from build123d import *

# Parameters (mm, degrees)
F0_W     = 75.653017
F0_H     = 55.848565
F1_DEPTH = 25.4
F2_SIZE  = 5.08
F4_DEPTH = 25.4


with BuildPart() as f1:
    # F0 (on Top) → F1 (new body)
    with BuildSketch(Plane.XY):
        with Locations((37.826508, 27.924283)):
            Rectangle(F0_W, F0_H)
    extrude(amount=-F1_DEPTH)

    # F2
    f2_edges = [f1.edges().sort_by_distance(p)[0] for p in [
        (0, 27.924282, 0),
        (37.826508, 0, 0),
        (75.653017, 27.924282, 0),
        (37.826508, 55.848565, 0),
    ]]
    chamfer(f2_edges, length=F2_SIZE)

    # F3 (on Top) → F4 (join)
    with BuildSketch(Plane.XY):
        Polygon((58.621187, 18.220101), (58.621187, 39.608911), (50.699413, 39.608911), (50.699413, 26.14188), (28.518412, 26.14188), (28.518412, 39.608911), (19.408364, 39.608911), (19.408364, 18.220101), align=None)
    extrude(amount=F4_DEPTH)


solid = f1.part
Verification items for the finished model (mm, model axes). A direction names the side the tool comes from. Give positions to 0.01 mm unless a question says otherwise; leave off trailing zeros. Order: outer loops, then holes, each group sorted by start corner. A loop starts at its lowest first (then second) coordinate and runs counter-clockwise, first axis right, second up. Notation, with made-up numbers: M -38,45 L -17,45 A29 cw -17,77 Z; hole C 34,13.25 d3. An arc over 180 degrees is marked long. Use one line per item in the form item = value. Start each with the question number.
Q1. Section check D-D (y = 30.5). Enter the section's corners in (x, z).
Q2. Section check C-C (z = 16.5). Enter the section's corners in (x, y), then the cut area to 3 significant figures.
Q3. Section check B-B (y = 22.5). Enter the section's corners in (x, z), then the cut area to 3 significant figures.
Q4. Go/stop test with flat-tipped pins: pin 1 Ø17 at (y, z) = (28.5, 8) entering from -X; pin 2 Ø6.5 at (y, z) = (26, 16.5) entering from +X; pin 3 Ø10 at (x, z) = (25.5, 14.5) entering from +Y. Record where each tip stops, or that it passes through.
Q5. Mould release check, pull along X, two halves, no side actions. Record for faces 1 (the flat face through (37.3, 53.27, -2.5)), 2 (the flat face through (40, 26.142, 13)), 3 (the flat face through (73.077, 27.533, -2.504)), 4 (the flat face through (50.699, 33, 13)): +X half, -X half, draft (parallel to the pull), parting line (faces both ways), or undercut.
Q6. Scan lines: line 1 along X through (y, z) = (36, 14.5); line 2 along Z through (x, y) = (69.5, 43); line 3 along X through (y, z) = (20, 2.5). Record each from-to range of solid material in increasing order. Write a range as [from, to].
Q7. Access from +Z, -Z, +X, -X, +Y, -Y to the whole of each face (thin tool, end or side, straight path). Record for faces 5 (the flat face through (39, 18.22, 13)), 6 (the flat face through (55, 39.609, 13)), 7 (the flat face through (28.518, 33, 13)).
Q8. Section check A-A (x = 30). Enter the section's corners in (y, z).
Evaluation:
q1.outline = M 0,-25.4 L 75.65,-25.4 L 75.65,-5.08 L 70.57,0 L 58.62,0 L 58.62,25.4 L 50.7,25.4 L 50.7,0 L 28.52,0 L 28.52,25.4 L 19.41,25.4 L 19.41,0 L 5.08,0 L 0,-5.08 Z
q2.outline = M 19.41,18.22 L 58.62,18.22 L 58.62,39.61 L 50.7,39.61 L 50.7,26.14 L 28.52,26.14 L 28.52,39.61 L 19.41,39.61 Z
q2.area = 540 mm2
q3.outline = M 0,-25.4 L 75.65,-25.4 L 75.65,-5.08 L 70.57,0 L 58.62,0 L 58.62,25.4 L 19.41,25.4 L 19.41,0 L 5.08,0 L 0,-5.08 Z
q3.area = 2,890 mm2
q4.pin_1 = 4.58
q4.pin_2 = 58.62
q4.pin_3 = 39.61
q5.face_1 = draft
q5.face_2 = undercut
q5.face_3 = +X half
q5.face_4 = undercut
q6.line_1 = [19.41, 28.52], [50.7, 58.62]
q6.line_2 = [-25.4, 0]
q6.line_3 = [19.41, 58.62]
q7.face_5 = +Z, +X, -X, -Y
q7.face_6 = +Z, +X, -X, +Y
q7.face_7 = +Z, +Y
q8.outline = M 0,-25.4 L 55.85,-25.4 L 55.85,-5.08 L 50.77,0 L 26.14,0 L 26.14,25.4 L 18.22,25.4 L 18.22,0 L 5.08,0 L 0,-5.08 Z
